The listing builds one solid part. Answer for the finished solid, in the listing's coordinates (mm). A direction names the side the tool comes from. Round coordinates to 2 decimals unless told otherwise and drop trailing zeros. Loops run counter-clockwise (first coordinate to the right, second up) from the corner with the lowest first, then second, coordinate; pieces in that order, holes last. Notation, with made-up numbers: M -6.75,-33 L 6.25,-33 A15 cw 6.25,-25 Z; hole C -21.5,65.5 d4. An arc over 180 degrees is marked long. Put each result on its own line as item: value. Start each with the question number.
(1) Flat-ended cylindrical pins translate along their axes: P1, Ø5, axis at x = 0.5, z = 20.5, coming from the -Y side; P2, Ø1.5, axis at x = -13.5, y = 6, coming from the -Z side; P3, Ø2.5, axis at x = -5.5, z = 26.5, coming from the +Y side. Find the tip coordinate at first contact, or state that the pin passes through.
(2) Straight lines are drawn through the part: line 1 (X direction, y = 6, z = 5); line 2 (Y direction, x = -11.75, z = 15.5); line 3 (X direction, y = 6.75, z = -4). For each, find the intervals that lie inside material, in ascending order.
(3) Section D-D, the plane z = 4 is taken. Determine the outline of the cut face in (x, y).
(4) Section C-C, the plane y = 3.5 is taken. Determine the outline of the cut face in (x, z).
(5) Which of the six approach directions +Z, -Z, +X, -X, +Y, -Y give full straight-line access (tool end or side, diameter ignored) to faces 1 (the face through (-5, 7.5, 3)), 2 (the face through (-5, -1, 5)), 3 (the face through (-7.5, 5, 26)), 4 (the face through (-10, 7.718, 16)), 5 (the face through (-10, 2.718, 16))?
(6) Section B-B, the plane x = -6.75 is taken. Determine the outline of the cut face in (y, z), then the cut area to 3 significant figures.
(7) Section A-A, the plane z = 19 is taken. Determine the outline of the cut face in (x, y), then the cut area to 3 significant figures.
```python
from build123d import *

# Parameters (mm, degrees)
F0_W     = 5
F0_H     = 5
F1_DEPTH = 10
F2_DEPTH = 20
F3_W     = 5
F3_H     = 5
F4_DEPTH = 20
F5_W     = 5
F5_H     = 4.782355
F6_DEPTH = 20


with BuildPart() as f1:
    # F0 (on Top) → F1 (new body)
    with BuildSketch(Plane.XY):
        Polygon((-5, -5), (5, -5), (5, 0), (0, 0), (0, 5), (-5, 5), align=None)
        with Locations((2.5, 2.5)):
            Rectangle(F0_W, F0_H)
    extrude(amount=F1_DEPTH)

    # F0 (on Top) → F2 (join)
    with BuildSketch(Plane.XY):
        Polygon((5, 5), (5, 0), (10, 0), (10, 10), (0, 10), (0, 5), align=None)
        with Locations((2.5, 2.5)):
            Rectangle(F0_W, F0_H)
    extrude(amount=F2_DEPTH)



with BuildPart() as f4:
    # F3 (on face) → F4 (new body)
    with BuildSketch(Plane(origin=(0, 0, 0), x_dir=(0, -1, 0), z_dir=(-1, 0, 0))):
        with Locations((-5.217645, 15.978696)):
            Rectangle(F3_W, F3_H)
    extrude(amount=F4_DEPTH)


with BuildPart() as f1_1:
    add(f1.part)

    add(f4.part)  # F6 merges F4
    # F5 (on face) → F6 (join, symmetric)
    with BuildSketch(Plane(origin=(0, 0, 13.478696), x_dir=(1, 0, 0), z_dir=(0, 0, -1))):
        with Locations((-5, -5.108823)):
            Rectangle(F5_W, F5_H)
    extrude(amount=F6_DEPTH, both=True)


solid = f1_1.part
```
Recorded:
1. P1: stops at y = 0
1. P2: stops at z = 13.48
1. P3: stops at y = 7.5
2. line 1: x = -7.5 to -2.5, 0 to 10
2. line 2: y = 2.72 to 7.72
2. line 3: x = -7.5 to -2.5
3. outline: M -7.5,2.72 L -5,2.72 L -5,-5 L 5,-5 L 5,0 L 10,0 L 10,10 L 0,10 L 0,5 L -2.5,5 L -2.5,7.5 L -7.5,7.5 Z
4. outline: M -20,13.48 L -7.5,13.48 L -7.5,-6.52 L -2.5,-6.52 L -2.5,0 L 10,0 L 10,20 L 0,20 L 0,18.48 L -2.5,18.48 L -2.5,33.48 L -7.5,33.48 L -7.5,18.48 L -20,18.48 Z; hole M -2.5,10 L 0,10 L 0,13.48 L -2.5,13.48 Z
5. face 1: -Z, -X, +Y
5. face 2: +Z, -Z, -X, -Y
5. face 3: +Z, -X, +Y, -Y
5. face 4: +Z, -Z, -X, +Y
5. face 5: +Z, -X, -Y
6. outline: M 2.72,-6.52 L 7.5,-6.52 L 7.5,13.48 L 7.72,13.48 L 7.72,18.48 L 7.5,18.48 L 7.5,33.48 L 2.72,33.48 Z
6. area: 192 mm²
7. outline: M -7.5,2.72 L -2.5,2.72 L -2.5,7.5 L -7.5,7.5 Z; M 0,0 L 10,0 L 10,10 L 0,10 Z
7. area: 124 mm²
